Part model, mm, in its own coordinate system. Give positions to 0.01 mm unless a question says otherwise; leave off trailing zeros. Write each loop counter-clockwise with the first axis right and the second up, starting at its lowest first coordinate (ties: lowest second). Pieces come first, ordered by that corner, then holes. Notation, with made-up numbers: (-24, 22.5) - (-7, 22.5) arc R18 cw to (-7, 47.5) - close; hole circle Ø2 at (61.5, -36.75). An arc over 180 degrees is marked (long way). Answer in a Markdown table with one row per item. Add a question column.
1. Band-saw the part on B-B on y = 50. Write the cut outline in (x, z).
2. Drop flat-ended pins along their axis: pin 1 Ø4.5 at (x, y) = (10, 50) entering from -Z (1 decimal); pin 2 Ø1.5 at (y, z) = (26, 1.5) entering from +X. Give the stop position or say it passes through.
3. Band-saw the part on C-C on z = 2.7. Write the cut outline in (x, y).
4. Band-saw the part on A-A on x = 30. Write the cut outline in (y, z), plus the area to 3 significant figures.
5. Pull direction Y, two halves, no side cores. Call faces 1 (the cylindrical face through (9.46, 52.44, 1.97)), 2 (the flat face through (23, 24, 0)), 3 (the flat face through (40, 40, 2)), 4 (the flat face through (30, 0, 2)): released by +Y, released by -Y, zero draft, split by the parting line, or undercut.
6. Band-saw the part on D-D on x = 10. Write the cut outline in (y, z).
7. Probe line 1 along Y through (x, z) = (10, 2.8); line 2 along Y through (x, z) = (12, 2.85); line 3 along X through (y, z) = (11.5, 0.6). List the from-to ranges inside material, lowest first.
Autodesk Inventor part; units mm, degrees
ref_plane "YZ Plane" through (0, 0, 0) normal (1, 0, 0) x (0, 1, 0)
ref_plane "XZ Plane" through (0, 0, 0) normal (0, 1, 0) x (-1, 0, 0)
ref_plane "XY Plane" through (0, 0, 0) normal (0, 0, 1) x (1, 0, 0)
sketch "Boceto1" plane through (0, 0, 0) normal (0, 0, 1) x (1, 0, 0)
  line L0 (190.1282, 320.5488) -> (475.893, 320.5488) construction
  line L1 (475.893, 320.5488) -> (475.893, 34.784) construction
  line L2 (475.893, 34.784) -> (190.1282, 34.784) construction
  line L3 (190.1282, 34.784) -> (190.1282, 320.5488) construction
  line L4 (0, 0) -> (0, 60)
  line L5 (0, 0) -> (60, 0)
  line L6 (60, 0) -> (60, 20)
  line L7 (60, 20) -> (20, 60)
  line L8 (20, 60) -> (0, 60)
  circle A0 centre (10, 50) radius 2.5
  circle A1 centre (10, 30) radius 2.5
  circle A2 centre (10, 10) radius 2.5
  circle A3 centre (30, 10) radius 2.5
  circle A4 centre (50, 10) radius 2.5
  point P0 (0, 30)
  point P1 (30, 0)
  dimension "d3" = 60
  dimension "d4" = 60
  dimension "d5" = 20
  dimension "d6" = 20
  dimension "d7" = 5
  dimension "d10" = 20
  dimension "d19" = 20
extrude "Extrusión1" add sketch "Boceto1" along normal blind 4
properties part number "LPlate" material "Aluminio 6061"
Values:
| question | item | result |
|---|---|---|
| 1 | outline | (0, 0) - (7.5, 0) - (7.5, 4) - (0, 4) - close; (12.5, 0) - (30, 0) - (30, 4) - (12.5, 4) - close |
| 2 | pin 1 | passes through |
| 2 | pin 2 | stops at x = 54.75 |
| 3 | outline | (0, 0) - (60, 0) - (60, 20) - (20, 60) - (0, 60) - close; hole circle Ø5 at (10, 10); hole circle Ø5 at (10, 30); hole circle Ø5 at (10, 50); hole circle Ø5 at (30, 10); hole circle Ø5 at (50, 10) |
| 4 | outline | (0, 0) - (7.5, 0) - (7.5, 4) - (0, 4) - close; (12.5, 0) - (50, 0) - (50, 4) - (12.5, 4) - close |
| 4 | area | 180 mm² |
| 5 | face 1 | undercut |
| 5 | face 2 | zero draft |
| 5 | face 3 | released by +Y |
| 5 | face 4 | released by -Y |
| 6 | outline | (0, 0) - (7.5, 0) - (7.5, 4) - (0, 4) - close; (12.5, 0) - (27.5, 0) - (27.5, 4) - (12.5, 4) - close; (32.5, 0) - (47.5, 0) - (47.5, 4) - (32.5, 4) - close; (52.5, 0) - (60, 0) - (60, 4) - (52.5, 4) - close |
| 7 | line 1 | y = 0 to 7.5, 12.5 to 27.5, 32.5 to 47.5, 52.5 to 60 |
| 7 | line 2 | y = 0 to 8.5, 11.5 to 28.5, 31.5 to 48.5, 51.5 to 60 |
| 7 | line 3 | x = 0 to 8, 12 to 28, 32 to 48, 52 to 60 |
